Build history of the part. All positions in model axes, mm. A direction names the side the tool comes from. Coordinates: 2 decimals unless noted, no trailing zeros. Write each question's results on one line, items separated by ' | '.
Autodesk Fusion 360 part; units mm, degrees
sketch "Sketch1" plane through (0, 0, 0) normal (0, 0, 1) x (1, 0, 0)
  line L0 (0, 0) -> (320, 0)
  line L1 (320, 0) -> (320, 100)
  line L2 (320, 100) -> (0, 100)
  line L3 (0, 100) -> (0, 0)
  dimension "d1" = 320
  dimension "d2" = 100
extrude "Extrude1" add sketch "Sketch1" along normal blind 10
sketch "Sketch2" plane through (0, 0, 10) normal (0, 0, 1) x (-1, 0, 0)
  line L0 (0, -100) -> (0, 0)
  line L1 (0, 0) -> (-320, 0)
  line L2 (-320, 0) -> (-320, -100)
  line L3 (-320, -100) -> (0, -100)
  circle A0 centre (-11, -90) radius 2.25
  circle A1 centre (-309, -90) radius 2.25
  circle A2 centre (-11, -80) radius 2.25
  circle A3 centre (-309, -80) radius 2.25
  circle A4 centre (-11, -70) radius 2.25
  circle A5 centre (-11, -60) radius 2.25
  circle A6 centre (-309, -70) radius 2.25
  circle A7 centre (-309, -60) radius 2.25
  dimension "d5" = 4.5
  dimension "d6" = 4.5
  dimension "d7" = 298
  dimension "d8" = 11
  dimension "d9" = 10
  dimension "d10" = 4.5
  dimension "d11" = 4.5
  dimension "d13" = 4.5
  dimension "d14" = 4.5
  dimension "d16" = 4.5
  dimension "d17" = 4.5
extrude "Extrude2" cut sketch "Sketch2" against normal blind 30 contours A0 | A1 | A2 | A3 | A4 | A5 | A6 | A7
sketch "Sketch3" plane through (0, 0, 10) normal (0, 0, 1) x (-1, 0, 0)
  circle A0 centre (-309, -80) radius 2.25
  circle A1 centre (-11, -80) radius 2.25
  circle A2 centre (-11, -70) radius 2.25
  circle A3 centre (-309, -70) radius 2.25
  circle A4 centre (-309, -90) radius 2.25
  circle A5 centre (-11, -90) radius 2.25
  circle A6 centre (-11, -60) radius 2.25
  circle A7 centre (-309, -60) radius 2.25
  line L0 (0, -100) -> (0, 0)
  line L1 (0, 0) -> (-320, 0)
  line L2 (-320, 0) -> (-320, -100)
  line L3 (-320, -100) -> (0, -100)
  circle A8 centre (-11, -90) radius 4
  dimension "d23" = 8
extrude "Extrude3" cut sketch "Sketch3" against normal blind 3.5 contours A8
pattern_linear "R-Pattern1" count 4 spacing 10 along (0, -1, 0) count 2 spacing 298 along (1, 0, 0) of "Extrude3"
sketch "Sketch4" plane through (0, 0, 10) normal (0, 0, 1) x (-1, 0, 0)
  circle A0 centre (-309, -60) radius 4
  circle A1 centre (-309, -70) radius 4
  circle A2 centre (-309, -80) radius 4
  circle A3 centre (-309, -90) radius 4
  circle A4 centre (-11, -60) radius 4
  circle A5 centre (-11, -70) radius 4
  circle A6 centre (-11, -80) radius 4
  circle A7 centre (-11, -90) radius 4
  line L0 (0, -100) -> (0, 0)
  line L1 (0, 0) -> (-320, 0)
  line L2 (-320, 0) -> (-320, -100)
  line L3 (-320, -100) -> (0, -100)
  line L4 (-317, -3) -> (-3, -3)
  line L5 (-3, -3) -> (-3, -97)
  line L6 (-3, -97) -> (-317, -97)
  line L7 (-317, -97) -> (-317, -3)
extrude "Extrude4" add sketch "Sketch4" along normal blind 5 contours L0 L1 L2 L3
sketch "Sketch5" plane through (0, 0, 10) normal (0, 0, 1) x (-1, 0, 0)
  line L0 (-3, -97) -> (-3, -3)
  line L1 (-3, -3) -> (-317, -3)
  line L2 (-317, -3) -> (-317, -97)
  line L3 (-317, -97) -> (-3, -97)
  circle A0 centre (-309, -60) radius 4
  circle A1 centre (-309, -70) radius 4
  circle A2 centre (-309, -80) radius 4
  circle A3 centre (-309, -90) radius 4
  circle A4 centre (-11, -60) radius 4
  circle A5 centre (-11, -70) radius 4
  circle A6 centre (-11, -80) radius 4
  circle A7 centre (-11, -90) radius 4
  circle A8 centre (-25, -50) radius 2.075
  circle A9 centre (-25, -25) radius 2.075
  circle A10 centre (-295, -50) radius 2.075
  circle A11 centre (-295, -25) radius 2.075
  dimension "d32" = 4.15
  dimension "d33" = 4.15
  dimension "d34" = 4.15
  dimension "d35" = 4.15
extrude "Extrude5" add sketch "Sketch5" along normal blind 3 contours A8 | A9 | A10 | A11
sketch "Sketch6" plane through (0, 0, 10) normal (0, 0, 1) x (-1, 0, 0)
  circle A0 centre (-295, -25) radius 2.075
  circle A1 centre (-25, -50) radius 2.075
  circle A2 centre (-295, -50) radius 2.075
  circle A3 centre (-25, -25) radius 2.075
  line L0 (-3, -97) -> (-3, -3)
  line L1 (-3, -3) -> (-317, -3)
  line L2 (-317, -3) -> (-317, -97)
  line L3 (-317, -97) -> (-3, -97)
  circle A4 centre (-309, -60) radius 4
  circle A5 centre (-309, -70) radius 4
  circle A6 centre (-309, -80) radius 4
  circle A7 centre (-309, -90) radius 4
  circle A8 centre (-11, -60) radius 4
  circle A9 centre (-11, -70) radius 4
  circle A10 centre (-11, -80) radius 4
  circle A11 centre (-11, -90) radius 4
  circle A12 centre (-45, -50) radius 2.075
  circle A13 centre (-45, -25) radius 2.075
  circle A14 centre (-275, -50) radius 2.075
  circle A15 centre (-275, -25) radius 2.075
  dimension "d38" = 4.15
  dimension "d39" = 4.15
  dimension "d40" = 4.15
  dimension "d41" = 4.15
extrude "Extrude6" cut sketch "Sketch6" against normal blind 3 contours A12 | A13 | A14 | A15
extrude "Extrude7" cut 1 faces at (212.3333, 1, 15) along direction (0, 0, -1) blind 15
extrude "Extrude8" cut 4 faces at (24.3391, 50.0023, 13) (25.1539, 24.4763, 13) (295.5715, 25.5958, 13) (294.4285, 49.4042, 13) along direction (0, 0, -1) blind 6
Item 1: Drill centre lines: line 1 (Y direction, x = 45, z = 8.25) (3 decimals); line 2 (Y direction, x = 309, z = 2.5); line 3 (X direction, y = 79.5, z = 7.75). Where is each one in solid material? Low to high. Write a range as from..to.
Answer:
line 1: y = 3..22.925, 27.075..47.925, 52.075..97 | line 2: y = 3..57.75, 62.25..67.75, 72.25..77.75, 82.25..87.75, 92.25..97 | line 3: x = 3..7.03, 14.97..305.03, 312.97..317
Item 2: Pull direction Y, two halves, no side cores. Call faces 3 (the flat face through (307, 62, 6.5)), 4 (the flat face through (158, 97, 5)), 5 (the flat face through (158, 51, 0)): released by +Y, released by -Y, zero draft, split by the parting line, or undercut.
Answer:
face 3: undercut | face 4: released by +Y | face 5: zero draft
Item 3: Tool access for faces 1 (the cylindrical face through (11.867, 73.905, 8.274)), 2 (the flat face through (158, 51, 10)): list every direction of +Z, -Z, +X, -X, +Y, -Y with a clear straight run to the whole face (end or side of a thin tool).
Answer:
face 1: +Z | face 2: +Z, +X, -X, +Y, -Y
Item 4: Pin check, flat tips, straight feed: pin 1 (2 mm diameter, centred on x = 24.5, y = 51, fed in from +Z); pin 2 (2 mm diameter, centred on x = 295.5, y = 49.5, fed in from +Z); pin 3 (2.5 mm diameter, centred on x = 13, y = 69, fed in from +Z). Stop position of each tip, or through.
Answer:
pin 1: stops at z = 10 | pin 2: stops at z = 7 | pin 3: stops at z = 6.5
